Here's how the part is built. I have some questions about the finished solid (model axes, mm). A direction names the side the tool comes from. Round coordinates to 2 decimals unless told otherwise and drop trailing zeros. Order: outer loops, then holes, each group sorted by start corner. A loop starts at its lowest first (then second) coordinate and runs counter-clockwise, first axis right, second up. Notation, with made-up numbers: (-5.5, 78) - (36.5, 78) arc R17 cw to (36.5, 91) - close; hole circle Ø6 at (13.5, -7). An arc over 180 degrees is marked (long way). One line per item, written item: value.
from build123d import *

# Parameters (mm, degrees)
SKETCH1_W           = 45.72
SKETCH1_H           = 22.86
SKETCH1_R           = 8.44
BOSS_EXTRUDE1_DEPTH = 6.35
SKETCH2_W           = 12.7
SKETCH2_H           = 3.81
CUT_EXTRUDE1_DEPTH  = 5.08
BOSS_EXTRUDE2_DEPTH = 2.54
SKETCH4_W           = 45.72
SKETCH4_H           = 2.032
BOSS_EXTRUDE3_DEPTH = 2.54
SKETCH5_R           = 2.54
CUT_EXTRUDE2_DEPTH  = 52.883813468


with BuildPart() as part:
    # Sketch1 → Boss-Extrude1 (new body)
    with BuildSketch(Plane.XY):
        with Locations((22.86, 11.43)):
            Rectangle(SKETCH1_W, SKETCH1_H)
        with Locations((9.906, 12.446)):
            Circle(SKETCH1_R, mode=Mode.SUBTRACT)
        with Locations((35.814, 12.446)):
            Circle(SKETCH1_R, mode=Mode.SUBTRACT)
        with BuildLine():
            Line((19.431, 7.62), (26.289, 7.62))
            ThreePointArc((26.289, 7.62), (28.829, 5.08), (26.289, 2.54))
            Line((26.289, 2.54), (19.431, 2.54))
            ThreePointArc((19.431, 2.54), (16.891, 5.08), (19.431, 7.62))
        make_face(mode=Mode.SUBTRACT)
    extrude(amount=BOSS_EXTRUDE1_DEPTH)

    # Sketch2 → Cut-Extrude1 (cut)
    with BuildSketch(Plane(origin=(0, 0, 0), x_dir=(-1, 0, 0), z_dir=(0, 0, -1))):
        with Locations((-22.86, 20.955)):
            Rectangle(SKETCH2_W, SKETCH2_H)
    extrude(amount=-CUT_EXTRUDE1_DEPTH, mode=Mode.SUBTRACT)

    # Sketch3 → Boss-Extrude2 (add)
    with BuildSketch(Plane(origin=(0, 22.86, 0), x_dir=(1, 0, 0), z_dir=(0, 1, 0))):
        Polygon((0, -6.35), (0, 8.89), (16.51, 8.89), (16.51, -5.08), (29.21, -5.08), (29.21, 8.89), (45.72, 8.89), (45.72, -6.35), align=None)
    extrude(amount=BOSS_EXTRUDE2_DEPTH)

    # Sketch4 → Boss-Extrude3 (add)
    with BuildSketch(Plane(origin=(0, 0, 0), x_dir=(-1, 0, 0), z_dir=(0, 0, -1))):
        with Locations((-22.86, 1.016)):
            Rectangle(SKETCH4_W, SKETCH4_H)
    extrude(amount=BOSS_EXTRUDE3_DEPTH)

    # Sketch5 → Cut-Extrude2 (cut, through all)
    with BuildSketch(Plane.XZ.offset(-22.86)):
        with Locations(Location((38.1, -5.08, 0), (0, 0, 270))):
            Circle(SKETCH5_R)
        with Locations(Location((7.62, -5.08, 0), (0, 0, 90))):
            Circle(SKETCH5_R)
    extrude(amount=-CUT_EXTRUDE2_DEPTH, mode=Mode.SUBTRACT)


solid = part.part
Q1. If we section it at B-B, the plane x = 22.5: Please give me the cut outline in (y, z).
Results list:
outline: (0, -2.54) - (2.03, -2.54) - (2.03, 0) - (2.54, 0) - (2.54, 6.35) - (0, 6.35) - close; (7.62, 0) - (19.05, 0) - (19.05, 5.08) - (25.4, 5.08) - (25.4, 6.35) - (7.62, 6.35) - close
Q2. If we section it at A-A, the plane z = -5.08: Please give me the cut outline in (x, y), then the cut area to 3 significant figures.
Results list:
outline: (0, 22.86) - (5.08, 22.86) - (5.08, 25.4) - (0, 25.4) - close; (10.16, 22.86) - (16.51, 22.86) - (16.51, 25.4) - (10.16, 25.4) - close; (29.21, 22.86) - (35.56, 22.86) - (35.56, 25.4) - (29.21, 25.4) - close; (40.64, 22.86) - (45.72, 22.86) - (45.72, 25.4) - (40.64, 25.4) - close
area: 58.1 mm²
Q3. Which directions (+Z, -Z, +X, -X, +Y, -Y) give clear straight access to the entire face, cutting with the end or side of a thin tool? Please do faces 1 (the flat face through (29.21, 24, 0)), 2 (the flat face through (23, 7.62, 3)), 3 (the cylindrical face through (5.1, 24.1, -5.4)), 4 (the flat face through (35.7, 22.86, -3.5)), 5 (the flat face through (23, 1, -2.54)).
Results list:
face 1: -Z, +Y
face 2: +Z, -Z
face 3: +Y, -Y
face 4: -Z, +X, -X
face 5: -Z, +X, -X, -Y
Q4. If I drill on line 1 along X through (y, z) = (23.95, -5.08); line 2 along Y through (x, z) = (5, -2.5); line 3 along X through (y, z) = (5, 2.5), over which ranges is the centre line in solid material (lowest first)?
Results list:
line 1: 0 to 5.08, 10.16 to 16.51, 29.21 to 35.56, 40.64 to 45.72
line 2: 0 to 2.03, 22.86 to 25.4
line 3: 0 to 5.93, 13.88 to 16.89, 28.83 to 31.84, 39.79 to 45.72
Q5. If we section it at D-D, the plane x = 38.1: Please give me the cut outline in (y, z), then the cut area to 3 significant figures.
Results list:
outline: (0, -2.54) - (2.03, -2.54) - (2.03, 0) - (4.32, 0) - (4.32, 6.35) - (0, 6.35) - close; (20.57, 0) - (22.86, 0) - (22.86, -2.54) - (25.4, -2.54) - (25.4, 6.35) - (20.57, 6.35) - close; (22.86, -8.89) - (25.4, -8.89) - (25.4, -7.62) - (22.86, -7.62) - close
area: 72.9 mm²
Q6. We'd pull the mould along X, two halves only. Please class faces 6 (the flat face through (45.72, 13, 2)), 7 (the cylindrical face through (40.62, 24.11, -4.75)), 8 (the cylindrical face through (16.89, 5.02, 3.13)), 9 (the flat face through (8, 24, -8.89)): released by +X, released by -X, zero draft, split by the parting line, or undercut.
Results list:
face 6: released by +X
face 7: undercut
face 8: undercut
face 9: zero draft
Q7. If we section it at C-C, the plane y = 15: Please give me the cut outline in (x, z).
Results list:
outline: (0, 0) - (1.86, 0) - (1.86, 6.35) - (0, 6.35) - close; (17.95, 0) - (27.77, 0) - (27.77, 6.35) - (17.95, 6.35) - close; (43.86, 0) - (45.72, 0) - (45.72, 6.35) - (43.86, 6.35) - close
Q8. Will these pins go through, and if not, where does the flat tip stop? pin 1 (15 mm diameter, centred on x = 35.814, y = 12.446, fed in from +Z); pin 2 (8 mm diameter, centred on x = 7.62, z = -5.08, fed in from -Y); pin 3 (10.5 mm diameter, centred on x = 20, y = 14.5, fed in from -Z); pin 4 (7 mm diameter, centred on x = 22.5, z = 1.5, fed in from +Y).
Results list:
pin 1: through
pin 2: y = 0
pin 3: z = 0
pin 4: y = 19.05
